The figure shows three views and two pictorial views of one solid part (mm, origin at its lowest corner). Answer the questions. Coordinates: 2 decimals unless noted, no trailing zeros. Loops run counter-clockwise (first coordinate to the right, second up) from the corner with the lowest first, then second, coordinate; pieces in that order, holes last. Notation, with made-up numbers: (-33.5, -20) - (7.5, -20) arc R11 ccw to (7.5, -4) - close; hole circle Ø8 at (-23, -25.75). An arc over 180 degrees is marked (long way). Return JSON: item names as keys, results as strings. Group by question number.
1. Find the intervals of material crossed by line 1 along Z through (x, y) = (3.5, 1.7) (1 decimal); line 2 along X through (y, z) = (2.4, 75); line 3 along Z through (x, y) = (47, 2.1) (1 decimal), in increasing order.
2. Section D-D (z = 28.5) is taken. Write down the section's boundary in (x, y) (3 decimals).
3. Section A-A (x = 10.16) is taken. Write down the section's boundary in (y, z) (3 decimals), and give its area (3 significant figures).
4. Section B-B (z = 10.16) is taken. Write down the section's boundary in (x, y) (3 decimals), and give its area (3 significant figures).
5. Each of these flat-tipped pins is pushed along its axis until it touches: P1, Ø2, axis at x = 3.25, z = 3.25, coming from the +Y side; P2, Ø1, axis at x = 10, y = 2.5, coming from the +Z side; P3, Ø1.6, axis at y = 2, z = 53, coming from the -X side. Where does it stop, or does it pass through?
6. Section C-C (y = 0.5) is taken. State how many separate pieces and enclosed holes the cut face has, and give its area (3 significant figures).
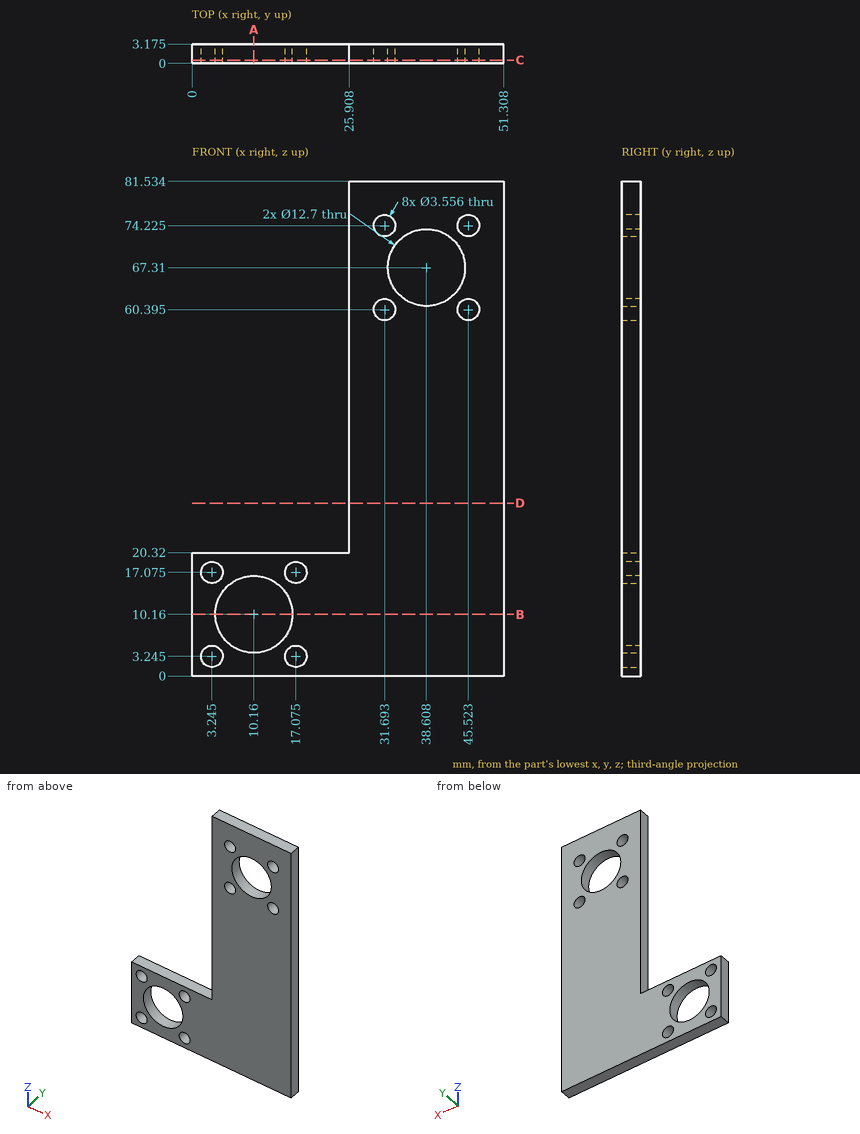
The answers:
{
 "1": {"line 1": "z = 0 to 1.5, 5 to 15.3, 18.8 to 20.3", "line 2": "x = 25.91 to 30.09, 33.29 to 43.92, 47.12 to 51.31", "line 3": "z = 0 to 59.4, 61.4 to 73.2, 75.2 to 81.5"},
 "2": {"outline": "(25.908, 0) - (51.308, 0) - (51.308, 3.175) - (25.908, 3.175) - close"},
 "3": {"outline": "(0, 0) - (3.175, 0) - (3.175, 3.81) - (0, 3.81) - close; (0, 16.51) - (3.175, 16.51) - (3.175, 20.32) - (0, 20.32) - close", "area": "24.2 mm2"},
 "4": {"outline": "(0, 0) - (3.81, 0) - (3.81, 3.175) - (0, 3.175) - close; (16.51, 0) - (51.308, 0) - (51.308, 3.175) - (16.51, 3.175) - close", "area": "123 mm2"},
 "5": {"P1": "passes through", "P2": "stops at z = 20.32", "P3": "stops at x = 25.91"},
 "6": {"separate pieces": "1", "enclosed holes": "10", "area": "2,260 mm2"}
}
